Model file for the job. Use its own axes, mm. Round coordinates to 2 decimals unless told otherwise and drop trailing zeros. Loops run counter-clockwise (first coordinate to the right, second up) from the corner with the lowest first, then second, coordinate; pieces in that order, holes last. Notation, with made-up numbers: M 42.5,43 L 92.5,43 A18 cw 92.5,48 Z; hole C -27,-39.5 d9. An arc over 180 degrees is marked long. Use a Markdown table: item, result. Add a question column.
Item 1: Saw through at B-B on y = 1.55. Write the cut outline in (x, z).
Item 2: Saw through at C-C on x = 259. Write the cut outline in (y, z), then the cut area to 3 significant figures.
Item 3: Pin check, flat tip, straight feed: P1, Ø4.5, axis at x = 276.5, z = 10, coming from the +Y side. Stop position of the tip, or through.
Item 4: Saw through at A-A on x = 340. Write the cut outline in (y, z), then the cut area to 3 significant figures.
Item 5: Wall check: L1, parallel to X at y = 4.5, z = 10; L2, parallel to Z at x = 309.5, y = 4.35; L3, parallel to Z at x = 194, y = 2.45. Give the ranges that are in metal, low to high. Write a range as from..to.
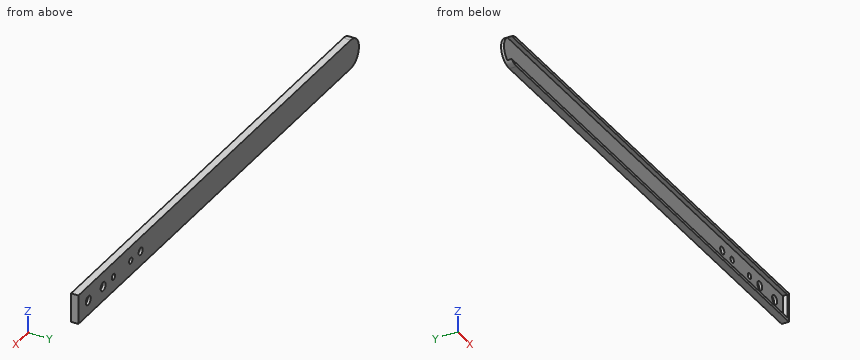
Autodesk Inventor part; units mm, degrees
ref_plane "YZ Plane" through (0, 0, 0) normal (1, 0, 0) x (0, 1, 0)
ref_plane "XZ Plane" through (0, 0, 0) normal (0, 1, 0) x (-1, 0, 0)
ref_plane "XY Plane" through (0, 0, 0) normal (0, 0, 1) x (1, 0, 0)
sketch "スケッチ1" plane through (0, 0, 0) normal (0, 0, 1) x (1, 0, 0)
  line L0 (0, 0) -> (352, 0)
  line L1 (352, 0) -> (352, 5)
  line L2 (352, 5) -> (0, 5)
  line L3 (0, 5) -> (0, 0)
  line L4 (0, 0) -> (6, 0)
  line L5 (0, 1) -> (0, 0)
  dimension "d0" = 352
  dimension "d1" = 5
extrude "押し出し1" add sketch "スケッチ1" along normal blind 20
sketch "スケッチ3" plane through (0, 0, 0) normal (-1, 0, 0) x (0, 0, 1)
  line L0 (0, 5) -> (0, 0)
  line L1 (0, 0) -> (20, 0)
  line L2 (20, 5) -> (20, 0)
  line L3 (0, 5) -> (20, 5)
  circle A0 centre (4, 2) radius 1.2
  circle A1 centre (16, 3) radius 1.2
  dimension "d14" = 2.4
  dimension "d15" = 2.4
  dimension "d16" = 3
  dimension "d17" = 4
  dimension "d18" = 4
  dimension "d19" = 3
extrude "押し出し3" cut sketch "スケッチ3" against normal blind 6 contours A0 | A1
sketch "スケッチ4" plane through (0, 0, 0) normal (0, -1, 0) x (1, 0, 0)
  line L0 (0, 0) -> (352, 0)
  line L1 (352, 0) -> (352, 20)
  line L2 (0, 20) -> (352, 20)
  line L3 (0, 0) -> (0, 20)
  line L4 (2, 2) -> (350, 2)
  line L5 (350, 2) -> (350, 18)
  line L6 (350, 18) -> (2, 18)
  line L7 (2, 18) -> (2, 2)
  dimension "d22" = 2
  dimension "d23" = 2
  dimension "d24" = 2
  dimension "d25" = 2
extrude "押し出し4" cut sketch "スケッチ4" against normal blind 3 contours L7 L6 L5 L4
sketch "スケッチ6" plane through (0, 3, 0) normal (0, -1, 0) x (1, 0, 0)
  line L0 (350, 18) -> (350, 2)
  line L1 (2, 18) -> (350, 18)
  point P0 (0, 0)
  point P1 (340, 10)
  dimension "d35" = 10
  dimension "d36" = 8
  dimension "d37" = 16
hole "穴1" at (340, 3, 10) direction (0, 1, 0) diameter 6 end through all
sketch "スケッチ7" plane through (0, 3, 0) normal (0, -1, 0) x (1, 0, 0)
  circle A0 centre (340, 10) radius 3
  line L0 (340, 10) -> (322, 10)
  point P0 (0, 0)
  dimension "d38" = 18
hole "穴2" at (322, 3, 10) direction (0, 1, 0) diameter 6 end through all
sketch "スケッチ8" plane through (0, 3, 0) normal (0, -1, 0) x (1, 0, 0)
  circle A0 centre (322, 10) radius 3
  line L0 (322, 10) -> (309.5, 10)
  point P0 (0, 0)
  dimension "d46" = 12.5
hole "穴3" at (309.5, 3, 10) direction (0, 1, 0) diameter 4 end through all
sketch "スケッチ9" plane through (0, 3, 0) normal (0, -1, 0) x (1, 0, 0)
  circle A0 centre (309.5, 10) radius 2
  line L0 (309.5, 10) -> (288.5, 10)
  point P0 (0, 0)
  dimension "d54" = 21
hole "穴4" at (288.5, 3, 10) direction (0, 1, 0) diameter 4 end through all
sketch "スケッチ10" plane through (0, 3, 0) normal (0, -1, 0) x (1, 0, 0)
  circle A0 centre (288.5, 10) radius 2
  line L0 (288.5, 10) -> (276.5, 10)
  point P0 (0, 0)
  dimension "d62" = 12
hole "穴5" at (276.5, 3, 10) direction (0, 1, 0) diameter 5 end through all
sketch "スケッチ11" plane through (0, 0, 0) normal (0, 0, -1) x (-1, 0, 0)
  line L0 (0, 0) -> (-352, 0)
  line L1 (0, 5) -> (0, 0)
  line L2 (-352, 5) -> (0, 5)
  line L3 (-352, 5) -> (0, 5)
  line L4 (0, 0) -> (-12, 0)
  line L5 (-12, 0) -> (-12, 5)
  line L6 (-12, 5) -> (0, 5)
  line L7 (0, 5) -> (0, 0)
  dimension "d70" = 12
extrude "押し出し5" cut sketch "スケッチ11" against normal through all
fillet "フィレット1" radius 10 2 edges at (12, 2.5, 20) (12, 2.5, 0)
properties part number "arm1_L"
Entries:
| question | item | result |
|---|---|---|
| 1 | outline | M 16,2 A10 ccw 22,0 L 352,0 L 352,20 L 22,20 A10 ccw 16,18 L 350,18 L 350,2 Z |
| 2 | outline | M 0,0 L 5,0 L 5,20 L 0,20 L 0,18 L 3,18 L 3,2 L 0,2 Z |
| 2 | area | 52.0 mm2 |
| 3 | P1 | through |
| 4 | outline | M 0,0 L 5,0 L 5,7 L 3,7 L 3,2 L 0,2 Z; M 0,18 L 3,18 L 3,13 L 5,13 L 5,20 L 0,20 Z |
| 4 | area | 40.0 mm2 |
| 5 | L1 | 12..274, 279..286.5, 290.5..307.5, 311.5..319, 325..337, 343..352 |
| 5 | L2 | 0..8, 12..20 |
| 5 | L3 | 0..2, 18..20 |
